CAD build for the part. Positions are in the model's coordinates, mm. A direction names the side the tool comes from. Round coordinates to 2 decimals unless told otherwise and drop trailing zeros. Write each loop counter-clockwise with the first axis right and the second up, starting at its lowest first coordinate (ties: lowest second). Pieces come first, ordered by that corner, then holes. Notation, with made-up numbers: (49.25, 36.5) - (103.25, 36.5) arc R30 cw to (103.25, 63.5) - close; hole circle Ø9 at (3, -19.5). An arc over 180 degrees is marked (long way). Use one line per item in the form item = value. Start each with the question number.
Item 1: Band-saw the part on A-A, the plane x = -84.5. List the corners of the cut face in (y, z).
Item 2: Pin check, flat tips, straight feed: pin 1 (4.5 mm diameter, centred on x = -113.64, z = -47.07, fed in from +Y); pin 2 (1 mm diameter, centred on x = -74.5, y = 8, fed in from -Z); pin 3 (6 mm diameter, centred on x = -95, y = 8.5, fed in from +Z); pin 4 (4 mm diameter, centred on x = -51.27, z = -51.27, fed in from +Y). Stop position of each tip, or through.
Item 3: Pull direction X, two halves, no side cores. Call faces 1 (the cylindrical face through (0.74, 9.57, -69.18)), 2 (the cylindrical face through (-50.242, 9.569, -48.023)), 3 (the cylindrical face through (116.84, 6.26, -48.13)), 4 (the cylindrical face through (-48.584, 6.261, 116.652)): +X half, -X half, draft (parallel to the pull), parting line (faces both ways), or undercut.
Item 4: Band-saw the part on C-C, the plane x = 42.5. List the corners of the cut face in (y, z), and give its area (3 significant figures).
Item 5: Band-saw the part on B-B, the plane x = 92. List the corners of the cut face in (y, z).
Item 6: Tool access for faces 5 (the cylindrical face through (-112.512, 1.315, 24.984)), 6 (the cylindrical face through (48.584, 6.261, -116.652)), 7 (the cylindrical face through (-48.023, 9.569, 50.242)): list every direction of +Z, -Z, +X, -X, +Y, -Y with a clear straight run to the whole face (end or side of a thin tool).
Item 7: Drill centre lines: L1, parallel to X at y = 2.1, z = 0; L2, parallel to X at y = 10.75, z = 0; L3, parallel to Z at x = -43, y = 2. Where is each one in solid material? Low to high.
from build123d import *

# Parameters (mm, degrees)
BOSS_EXTRUDE1_DEPTH   = 12.7
SKETCH3_R             = 24.5745
CUT_EXTRUDE1_DEPTH    = 174.423960282
SKETCH5_R             = 51.3715
SKETCH5_R_2           = 46.5455
CUT_EXTRUDE2_DEPTH    = 2.794
SKETCH37_R            = 119.0625
SKETCH37_R_2          = 115.2525
CUT_EXTRUDE7_DEPTH    = 2.667
CIRPATTERN4_COUNT     = 8
F_8_32_TAPPED_HOLE1_D = 3.4544
CIRPATTERN5_COUNT     = 8


with BuildPart() as part:
    # Sketch1 → Boss-Extrude1 (new body)
    with BuildSketch(Plane(origin=(0, 0, 0), x_dir=(1, 0, 0), z_dir=(0, 1, 0))):
        with BuildLine():
            ThreePointArc((-31.793446259, 122.3), (-48.357791931, 116.746037126), (-63.997797892, 108.960520786))
            Line((-63.997797892, 108.960520786), (-108.960520786, 63.997797892))
            ThreePointArc((-108.960520786, 63.997797892), (-116.746037126, 48.357791931), (-122.3, 31.793446259))
            Line((-122.3, 31.793446259), (-122.3, -31.793446259))
            ThreePointArc((-122.3, -31.793446259), (-116.746037126, -48.357791931), (-108.960520786, -63.997797892))
            Line((-108.960520786, -63.997797892), (-63.997797892, -108.960520786))
            ThreePointArc((-63.997797892, -108.960520786), (-48.357791931, -116.746037126), (-31.793446259, -122.3))
            Line((-31.793446259, -122.3), (31.793446259, -122.3))
            ThreePointArc((31.793446259, -122.3), (48.357791931, -116.746037126), (63.997797892, -108.960520786))
            Line((63.997797892, -108.960520786), (108.960520786, -63.997797892))
            ThreePointArc((108.960520786, -63.997797892), (116.746037126, -48.357791931), (122.3, -31.793446259))
            Line((122.3, -31.793446259), (122.3, 31.793446259))
            ThreePointArc((122.3, 31.793446259), (116.746037126, 48.357791931), (108.960520786, 63.997797892))
            Line((108.960520786, 63.997797892), (63.997797892, 108.960520786))
            ThreePointArc((63.997797892, 108.960520786), (48.357791931, 116.746037126), (31.793446259, 122.3))
            Line((31.793446259, 122.3), (-31.793446259, 122.3))
        make_face()
    extrude(amount=BOSS_EXTRUDE1_DEPTH)

    # Sketch3 → Cut-Extrude1 (cut, through all)
    with BuildSketch(Plane(origin=(0, 12.7, 0), x_dir=(1, 0, 0), z_dir=(0, 1, 0))):
        with Locations(Location((0, 0, 0), (0, 0, 270))):
            Circle(SKETCH3_R)
    extrude(amount=-CUT_EXTRUDE1_DEPTH, mode=Mode.SUBTRACT)

    # Sketch5 → Cut-Extrude2 (cut)
    with BuildSketch(Plane(origin=(0, 12.7, 0), x_dir=(1, 0, 0), z_dir=(0, 1, 0))):
        with Locations(Location((0, 0, 0), (0, 0, 270))):
            Circle(SKETCH5_R)
        with Locations(Location((0, 0, 0), (0, 0, 270))):
            Circle(SKETCH5_R_2, mode=Mode.SUBTRACT)
    extrude(amount=-CUT_EXTRUDE2_DEPTH, mode=Mode.SUBTRACT)

    # Sketch23 → M8x1.25 Tapped Hole1 (revolve, cut)
    with BuildSketch(Plane(origin=(-72.5, 12.7, 0), x_dir=(0, 0, 1), z_dir=(1, 0, 0))):
        Polygon((0, 0), (0, 8.392926105), (3.4, 6.35), (3.4, 0), align=None)
    m8x1_25_tapped_hole1 = revolve(axis=Axis((-72.5, 19.05, 0), (0, -1, 0)), mode=Mode.SUBTRACT)

    # Sketch37 → Cut-Extrude7 (cut)
    with BuildSketch(Plane.XZ):
        with Locations(Location((0, 0, 0), (0, 0, 270))):
            Circle(SKETCH37_R)
        with Locations(Location((0, 0, 0), (0, 0, 270))):
            Circle(SKETCH37_R_2, mode=Mode.SUBTRACT)
    extrude(amount=-CUT_EXTRUDE7_DEPTH, mode=Mode.SUBTRACT)

    # CirPattern4: M8x1.25 Tapped Hole1 ×8 about axis
    cirpattern4_axis = Axis((0, 0, 0), (0, 1, 0))
    for i in range(1, CIRPATTERN4_COUNT):
        add(m8x1_25_tapped_hole1.rotate(cirpattern4_axis, i * 360 / CIRPATTERN4_COUNT), mode=Mode.SUBTRACT)

    # #8-32 Tapped Hole1 (through all)
    with Locations(Plane(origin=(0, 12.7, 0), x_dir=(1, 0, 0), z_dir=(0, 1, 0))):
        with Locations((-47.069870839, 113.636720559)):
            f_8_32_tapped_hole1 = Hole(F_8_32_TAPPED_HOLE1_D / 2)

    # CirPattern5: #8-32 Tapped Hole1 ×8 about axis
    cirpattern5_axis = Axis((0, 0, 0), (0, 1, 0))
    for i in range(1, CIRPATTERN5_COUNT):
        add(f_8_32_tapped_hole1.rotate(cirpattern5_axis, i * 360 / CIRPATTERN5_COUNT), mode=Mode.SUBTRACT)


solid = part.part
Determined:
q1.outline = (0, -88.46) - (12.7, -88.46) - (12.7, 88.46) - (0, 88.46) - (0, 83.88) - (2.67, 83.88) - (2.67, 78.38) - (0, 78.38) - (0, -78.38) - (2.67, -78.38) - (2.67, -83.88) - (0, -83.88) - close
q2.pin_1 = 12.7
q2.pin_2 = -98.96
q2.pin_3 = 80.96
q2.pin_4 = 5.51
q3.face_1 = undercut
q3.face_2 = undercut
q3.face_3 = +X half
q3.face_4 = -X half
q4.outline = (0, -119) - (12.7, -119) - (12.7, -28.86) - (9.91, -28.86) - (9.91, -18.98) - (12.7, -18.98) - (12.7, 18.98) - (9.91, 18.98) - (9.91, 28.86) - (12.7, 28.86) - (12.7, 119) - (0, 119) - (0, 111.22) - (2.67, 111.22) - (2.67, 107.13) - (0, 107.13) - (0, -107.13) - (2.67, -107.13) - (2.67, -111.22) - (0, -111.22) - close
q4.area = 2,950 mm²
q5.outline = (0, -80.96) - (12.7, -80.96) - (12.7, 80.96) - (0, 80.96) - (0, 75.58) - (2.67, 75.58) - (2.67, 69.42) - (0, 69.42) - (0, -69.42) - (2.67, -69.42) - (2.67, -75.58) - (0, -75.58) - close
q6.face_5 = -Y
q6.face_6 = -Z, +X, +Y, -Y
q6.face_7 = +Y
q7.L1 = -122.3 to -119.06, -115.25 to -24.57, 24.57 to 115.25, 119.06 to 122.3
q7.L2 = -122.3 to -75.9, -69.1 to -51.37, -46.55 to -24.57, 24.57 to 46.55, 51.37 to 69.1, 75.9 to 122.3
q7.L3 = -118.82 to -111.03, -106.93 to 106.93, 111.03 to 118.82
